Geometry: see drawing. Coordinates: mm, zero at the bounding-box minimum. A direction names the side the tool comes from. Round coordinates to 2 decimals unless told otherwise and drop trailing zeros. Loops run counter-clockwise (first coordinate to the right, second up) from the corner with the lowest first, then second, coordinate; pieces in that order, holes last. Notation, with made-up numbers: (-16, 31) - (27, 31) arc R28 cw to (27, 61) - close; hole circle Ø11 at (54, 19.5). An arc over 180 degrees is marked (long way). Use CSV: the item, a comma, the result in double quotes.
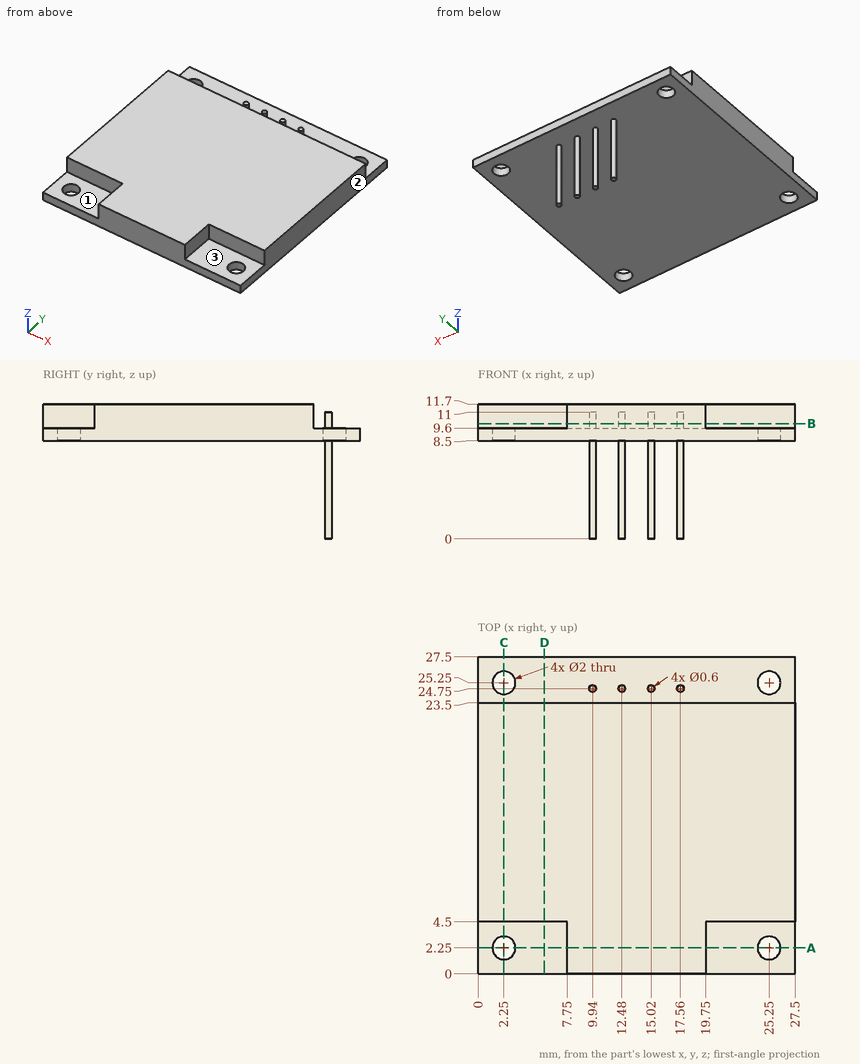
Item 1: Reachability of the marked faces 1, 2 and 3 from +Z, -Z, +X, -X, +Y, -Y: full face, straight path, thin tool, end or side. Return the list, or none.
Final values:
face 1,"+Z, -X, -Y"
face 2,"+Z, -Z, +X, +Y, -Y"
face 3,"+Z, +X, -Y"
Item 2: Material intervals for line 1 (Y direction, x = 25.25, z = 8.7); line 2 (Z direction, x = 5.5, y = 10.5), sorted ascending.
Final values:
line 1,"y = 0 to 1.25, 3.25 to 24.25, 26.25 to 27.5"
line 2,"z = 8.5 to 11.7"
Item 3: Section A-A on y = 2.25. Return the cut outline in (x, z).
Final values:
outline,"(0, 8.5) - (1.25, 8.5) - (1.25, 9.6) - (0, 9.6) - close; (3.25, 8.5) - (24.25, 8.5) - (24.25, 9.6) - (19.75, 9.6) - (19.75, 11.7) - (7.75, 11.7) - (7.75, 9.6) - (3.25, 9.6) - close; (26.25, 8.5) - (27.5, 8.5) - (27.5, 9.6) - (26.25, 9.6) - close"
Item 4: Section C-C on x = 2.25. Return the cut outline in (y, z).
Final values:
outline,"(0, 8.5) - (1.25, 8.5) - (1.25, 9.6) - (0, 9.6) - close; (3.25, 8.5) - (24.25, 8.5) - (24.25, 9.6) - (23.5, 9.6) - (23.5, 11.7) - (4.5, 11.7) - (4.5, 9.6) - (3.25, 9.6) - close; (26.25, 8.5) - (27.5, 8.5) - (27.5, 9.6) - (26.25, 9.6) - close"
Item 5: Section D-D on x = 5.75. Return the cut outline in (y, z).
Final values:
outline,"(0, 8.5) - (27.5, 8.5) - (27.5, 9.6) - (23.5, 9.6) - (23.5, 11.7) - (4.5, 11.7) - (4.5, 9.6) - (0, 9.6) - close"
Item 6: Section B-B on z = 10. Return the cut outline in (x, y).
Final values:
outline,"(0, 4.5) - (7.75, 4.5) - (7.75, 0) - (19.75, 0) - (19.75, 4.5) - (27.5, 4.5) - (27.5, 23.5) - (0, 23.5) - close; circle Ø0.6 at (9.94, 24.75); circle Ø0.6 at (12.48, 24.75); circle Ø0.6 at (15.02, 24.75); circle Ø0.6 at (17.56, 24.75)"
Item 7: Pin query (flat end, axial travel): P1, Ø1, axis at x = 9, y = 9.5, coming from the -Z side; P2, Ø1, axis at x = 8.5, z = 10.5, coming from the +Y side; P3, Ø1, axis at x = 12.5, z = 3.5, coming from the -Y side. Return the tip coordinate at first contact, or that it passes through.
Final values:
P1,"stops at z = 8.5"
P2,"stops at y = 23.5"
P3,"stops at y = 24.45"
